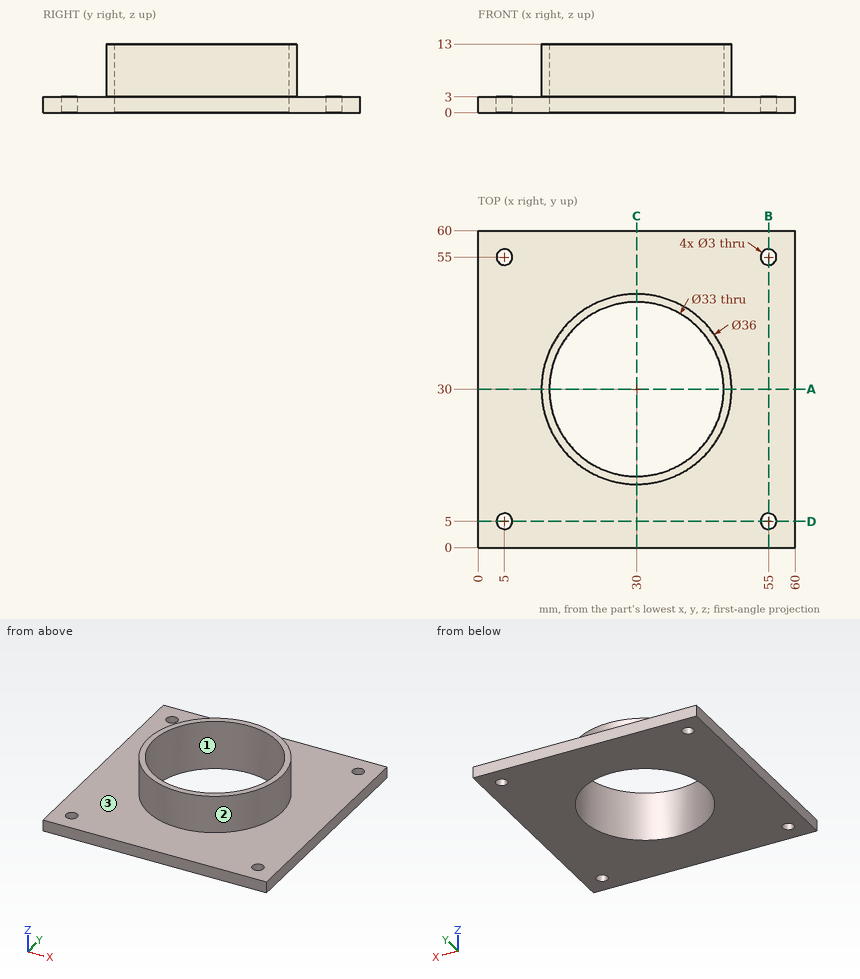
Answer from the drawing. Dimensions are ordinates in mm from the lowest x, y and z of the part. Give positions to 0.01 mm unless a question says otherwise; leave off trailing zeros. Write each loop counter-clockwise with the first axis right and the second up, starting at its lowest first coordinate (ties: lowest second). Pieces come first, ordered by that corner, then holes.
1) For a pull along X with two mould halves and no side action, classify the marked faces 1, 2 and 3 as pulls with the +X half, pulls with the -X half, needs draft (parallel to the pull), parting line crosses it, or undercut.
2) Section B-B (x = 55) is taken. Write down the section's boundary in (y, z), and give its area (3 significant figures).
3) Find the intervals of material crossed by L1, parallel to Y at x = 55, z = 2.4; L2, parallel to Y at x = 30, z = 5; L3, parallel to X at y = 4.5, z = 2.5, in increasing order.
4) Given P1, Ø5, axis at x = 5, y = 5, coming from the +Z side; P2, Ø2.5, axis at x = 5, y = 55, coming from the -Z side; P3, Ø5, axis at x = 36, y = 10, coming from the -Z side; P4, Ø1, axis at x = 23.5, z = 7, coming from the +Y side, each flat-ended and moving along its own axis, determine where each tip first touches the part or whether it passes through.
5) Section A-A (y = 30) is taken. Write down the section's boundary in (x, z), and give its area (3 significant figures).
Response:
1. face 1: undercut
1. face 2: parting line crosses it
1. face 3: needs draft
2. outline: (0, 0) - (3.5, 0) - (3.5, 3) - (0, 3) - close; (6.5, 0) - (53.5, 0) - (53.5, 3) - (6.5, 3) - close; (56.5, 0) - (60, 0) - (60, 3) - (56.5, 3) - close
2. area: 162 mm2
3. L1: y = 0 to 3.5, 6.5 to 53.5, 56.5 to 60
3. L2: y = 12 to 13.5, 46.5 to 48
3. L3: x = 0 to 3.59, 6.41 to 53.59, 56.41 to 60
4. P1: stops at z = 3
4. P2: passes through
4. P3: stops at z = 0
4. P4: stops at y = 46.97
5. outline: (0, 0) - (13.5, 0) - (13.5, 13) - (12, 13) - (12, 3) - (0, 3) - close; (46.5, 0) - (60, 0) - (60, 3) - (48, 3) - (48, 13) - (46.5, 13) - close
5. area: 111 mm2
